Job drawing, mm, ordinate dimensions from the low corner. One solid piece. Round coordinates to 2 decimals unless told otherwise and drop trailing zeros. Loops run counter-clockwise (first coordinate to the right, second up) from the corner with the lowest first, then second, coordinate; pieces in that order, holes last.
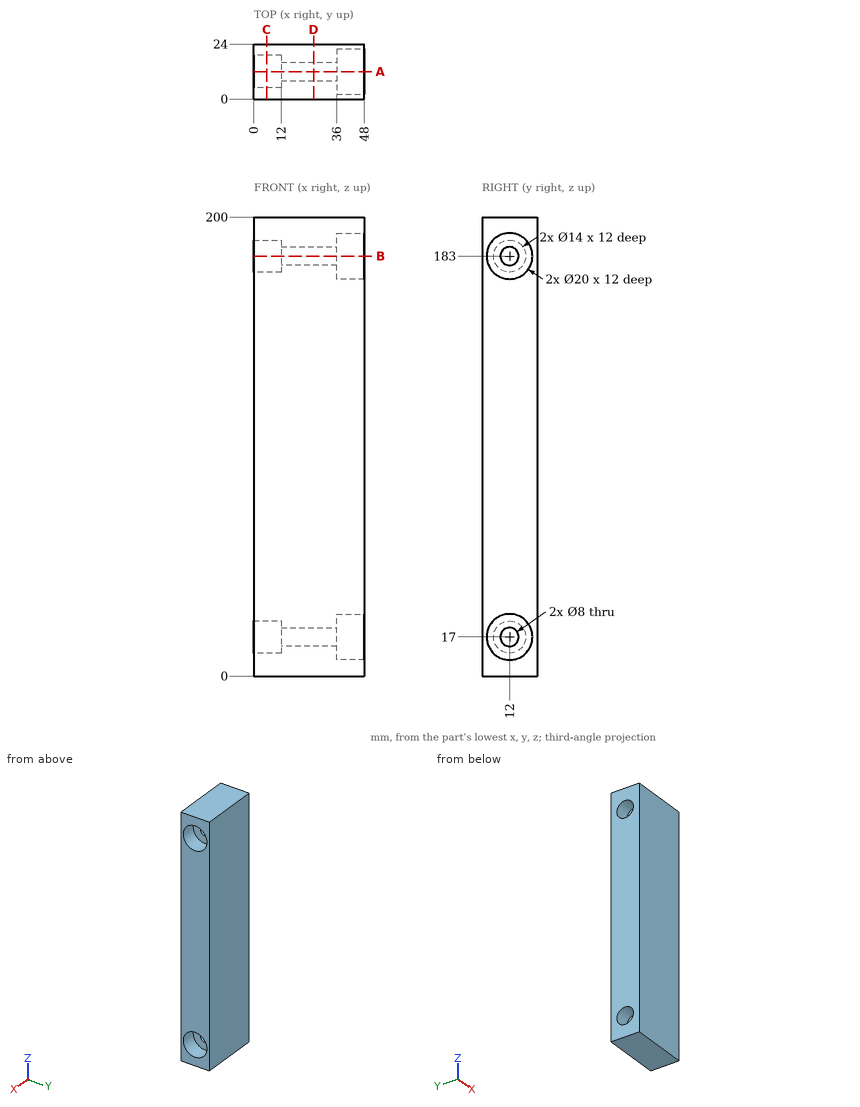
Item 1: Cut at D-D, the plane x = 26. Give the cut face in (y, z), plus the area to 3 significant figures.
Answers follow:
outline: (0, 0) - (24, 0) - (24, 200) - (0, 200) - close; hole circle Ø8 at (12, 17); hole circle Ø8 at (12, 183)
area: 4,700 mm2
Item 2: Probe line 1 (Y direction, x = 6, z = 17); line 2 (Z direction, x = 2, y = 15); line 3 (Z direction, x = 15, y = 14.25). List the from-to ranges inside material, lowest first.
Answers follow:
line 1: y = 0 to 5, 19 to 24
line 2: z = 0 to 10.68, 23.32 to 176.68, 189.32 to 200
line 3: z = 0 to 13.69, 20.31 to 179.69, 186.31 to 200
Item 3: Cut at B-B, the plane z = 183. Give the cut face in (x, y).
Answers follow:
outline: (0, 0) - (48, 0) - (48, 2) - (36, 2) - (36, 8) - (12, 8) - (12, 5) - (0, 5) - close; (0, 19) - (12, 19) - (12, 16) - (36, 16) - (36, 22) - (48, 22) - (48, 24) - (0, 24) - close
Item 4: Cut at A-A, the plane y = 12. Give the cut face in (x, z), plus the area to 3 significant figures.
Answers follow:
outline: (0, 0) - (48, 0) - (48, 7) - (36, 7) - (36, 13) - (12, 13) - (12, 10) - (0, 10) - close; (0, 24) - (12, 24) - (12, 21) - (36, 21) - (36, 27) - (48, 27) - (48, 173) - (36, 173) - (36, 179) - (12, 179) - (12, 176) - (0, 176) - close; (0, 190) - (12, 190) - (12, 187) - (36, 187) - (36, 193) - (48, 193) - (48, 200) - (0, 200) - close
area: 8,400 mm2
Item 5: Cut at C-C, the plane x = 5.5. Give the cut face in (y, z), plus the area to 3 significant figures.
Answers follow:
outline: (0, 0) - (24, 0) - (24, 200) - (0, 200) - close; hole circle Ø14 at (12, 17); hole circle Ø14 at (12, 183)
area: 4,490 mm2
Item 6: Flat gauge pins, fed straight in: P1, Ø4, axis at y = 14.5, z = 180.5, coming from the -X side; P2, Ø6, axis at y = 13.5, z = 15, coming from the +X side; P3, Ø6.5, axis at y = 12, z = 183, coming from the +X side. Where does each tip first touch, or does it go through?
Answers follow:
P1: stops at x = 12
P2: stops at x = 36
P3: passes through
